Check sheet for the modelled part. Datum: model origin and axes. Units: mm. A direction names the side the tool comes from. Coordinates: 2 decimals unless noted, no trailing zeros. Loops run counter-clockwise (first coordinate to the right, second up) from the corner with the lowest first, then second, coordinate; pieces in that order, holes last. Notation, with made-up numbers: (-10.5, -16.5) - (0.5, -16.5) arc R22 ccw to (0.5, 21.5) - close; hole circle Ø4 at (6, 30.25). An arc over 180 degrees is marked (long way). Use a Markdown table: item, result. Add a question column.
1) Tool access check on faces 5 (the flat face through (30.4, 19.9, 4.5)), 6 (the flat face through (-31, 18.5, 17)). Record the directions out of +Z, -Z, +X, -X, +Y, -Y that give a thin tool (end or side, any length) a straight path to the whole face; none if there is none.
2) Sectioned sample at B-B, the plane z = 18.75. Enter the section's corners in (x, y), then the cut area to 3 significant figures.
3) Sectioned sample at A-A, the plane x = 31. Enter the section's corners in (y, z).
4) Go/stop test with flat-tipped pins: P1, Ø2, axis at x = 21, z = 5.5, coming from the +Y side; P2, Ø0.9, axis at y = -11, z = 1.5, coming from the -X side; P3, Ø2, axis at x = -3.5, z = 5.5, coming from the -Y side. Record where each tip stops, or that it passes through.
5) Sectioned sample at C-C, the plane y = 15.5. Enter the section's corners in (x, z).
6) Draft check along X on faces 1 (the cylindrical face through (-36.1, 20.02, 26.14)), 2 (the flat face through (0, 41.5, 8)), 3 (the flat face through (37, 20, 18)), 4 (the cylindrical face through (14, -15.43, 1.52)). Enter one of: pulls with the +X half, pulls with the -X half, needs draft (parallel to the pull), parting line crosses it, or undercut.
7) Sectioned sample at D-D, the plane z = 13.75. Enter the section's corners in (x, y), then the cut area to 3 significant figures.
8) Thickness scan on line 1 (X direction, y = 20.6, z = 20); line 2 (X direction, y = 5, z = 12.25); line 3 (Y direction, x = -15.5, z = 1.8). Record the ranges inside material, lowest first.
from build123d import *

# Parameters (mm, degrees)
BOSS_EXTRUDE1_DEPTH     = 3
BOSS_EXTRUDE2_DEPTH     = 27
BOSS_EXTRUDE2_2_DEPTH   = 27
BOSS_EXTRUDE3_DEPTH     = 10
SKETCH4_W               = 26
SKETCH4_H               = 17
BOSS_EXTRUDE4_DEPTH     = 7
CUT_EXTRUDE1_DEPTH      = 80.342611502
SKETCH6_R               = 2.2
CUT_EXTRUDE2_DEPTH      = 61.811183182
SKETCH7_W               = 20
SKETCH7_H               = 7
CUT_EXTRUDE3_DEPTH      = 17
SKETCH8_R               = 12
SKETCH8_R_2             = 1.5
CUT_EXTRUDE4_DEPTH      = 61.557823607
SKETCH9_R               = 2.2
CUT_EXTRUDE5_DEPTH      = 59.139917441
FILLET1_R               = 7
FILLET2_R               = 3
CHAMFER1_SIZE           = 6
CUT_EXTRUDE6_DEPTH      = 61.557823607
CUT_EXTRUDE6_DEPTH_BACK = 61.557823607
FILLET3_R               = 1


with BuildPart() as part:
    # Sketch1 → Boss-Extrude1 (new body)
    with BuildSketch(Plane.XY):
        Polygon((-13, 21.5), (-13, 41.5), (13, 41.5), (13, 21.5), (22, 21.5), (22, -21.5), (-22, -21.5), (-22, 21.5), align=None)
    extrude(amount=BOSS_EXTRUDE1_DEPTH)



with BuildPart() as body_2:
    # Sketch2 → Boss-Extrude2 (new body)
    with BuildSketch(Plane(origin=(0, 0, 0), x_dir=(-1, 0, 0), z_dir=(0, 0, -1))):
        Polygon((37, 21.5), (22, 21.5), (22, -7.5), (25, -7.5), (25, 18.5), (37, 18.5), align=None)
    extrude(amount=-BOSS_EXTRUDE2_DEPTH)


with BuildPart() as body_3:
    # Sketch2 → Boss-Extrude2 2 (new body)
    with BuildSketch(Plane(origin=(0, 0, 0), x_dir=(-1, 0, 0), z_dir=(0, 0, -1))):
        Polygon((-37, 18.5), (-37, 21.5), (-22, 21.5), (-22, -7.5), (-25, -7.5), (-25, 18.5), align=None)
    extrude(amount=-BOSS_EXTRUDE2_2_DEPTH)


with BuildPart() as part_1:
    add(part.part)

    add(body_2.part)  # Boss-Extrude3 merges body 2

    add(body_3.part)  # Boss-Extrude3 merges body 3
    # Sketch3 → Boss-Extrude3 (add)
    with BuildSketch(Plane(origin=(0, 0, 0), x_dir=(-1, 0, 0), z_dir=(0, 0, -1))):
        Polygon((-25, 21.5), (-22, 24.5), (22, 24.5), (25, 21.5), align=None)
    extrude(amount=-BOSS_EXTRUDE3_DEPTH)

    # Sketch4 → Boss-Extrude4 (add)
    with BuildSketch(Plane.XY.offset(3)):
        with Locations((0, 33)):
            Rectangle(SKETCH4_W, SKETCH4_H)
    extrude(amount=BOSS_EXTRUDE4_DEPTH)

    # Sketch5 → Cut-Extrude1 (cut, through all)
    with BuildSketch(Plane(origin=(25, 0, 0), x_dir=(0, 0, -1), z_dir=(1, 0, 0))):
        Polygon((-27, 18.5), (-3, -7.5), (-27, -7.5), align=None)
    extrude(amount=-CUT_EXTRUDE1_DEPTH, mode=Mode.SUBTRACT)

    # Sketch6 → Cut-Extrude2 (cut, through all)
    with BuildSketch(Plane.XZ.offset(-18.5)):
        with Locations(Location((31, 20, 0), (0, 0, 270))):
            Circle(SKETCH6_R)
        with Locations(Location((-31, 20, 0), (0, 0, 180))):
            Circle(SKETCH6_R)
        Polygon((25, 0), (37, 10), (37, 0), align=None)
        Polygon((-37, 0), (-25, 0), (-37, 10), align=None)
    extrude(amount=-CUT_EXTRUDE2_DEPTH, mode=Mode.SUBTRACT)

    # Sketch7 → Cut-Extrude3 (cut)
    with BuildSketch(Plane(origin=(0, 41.5, 0), x_dir=(1, 0, 0), z_dir=(0, 1, 0))):
        with Locations((0, -3.5)):
            Rectangle(SKETCH7_W, SKETCH7_H)
    extrude(amount=-CUT_EXTRUDE3_DEPTH, mode=Mode.SUBTRACT)

    # Sketch8 → Cut-Extrude4 (cut, through all)
    with BuildSketch(Plane.XY.offset(3)):
        Circle(SKETCH8_R)
        with Locations((-15.5, 15.5)):
            Circle(SKETCH8_R_2)
        with Locations((15.5, 15.5)):
            Circle(SKETCH8_R_2)
        with Locations((15.5, -15.5)):
            Circle(SKETCH8_R_2)
        with Locations((-15.5, -15.5)):
            Circle(SKETCH8_R_2)
    extrude(amount=-CUT_EXTRUDE4_DEPTH, mode=Mode.SUBTRACT)

    # Sketch9 → Cut-Extrude5 (cut, through all)
    with BuildSketch(Plane.XY.offset(10)):
        with Locations((0, 31.5)):
            Circle(SKETCH9_R)
    extrude(amount=-CUT_EXTRUDE5_DEPTH, mode=Mode.SUBTRACT)

    # Fillet1
    fillet1_edges = [part_1.edges().sort_by_distance(p)[0] for p in [
        (13, 24.5, 5),
        (-13, 24.5, 5),
    ]]
    fillet(fillet1_edges, radius=FILLET1_R)

    # Fillet2
    fillet2_edges = [part_1.edges().sort_by_distance(p)[0] for p in [
        (13, 41.5, 5),
        (-13, 41.5, 5),
        (-37, 20, 10),
        (37, 20, 10),
        (-37, 20, 27),
        (37, 20, 27),
    ]]
    fillet(fillet2_edges, radius=FILLET2_R)

    # Chamfer1
    chamfer1_edges = [part_1.edges().sort_by_distance(p)[0] for p in [
        (22, -21.5, 1.5),
        (-22, -21.5, 1.5),
    ]]
    chamfer(chamfer1_edges, length=CHAMFER1_SIZE)

    # Sketch10 → Cut-Extrude6 (cut, two sides: drawn at the far end of the back side and taken through both)
    with BuildSketch(Plane.XY.offset(3).offset(-CUT_EXTRUDE6_DEPTH_BACK)):
        Polygon((22, -7.5), (25, -4.510011911), (25, -7.5), align=None)
        Polygon((-22, -7.5), (-25, -7.5), (-25, -4.510005014), align=None)
    extrude(amount=CUT_EXTRUDE6_DEPTH + CUT_EXTRUDE6_DEPTH_BACK, mode=Mode.SUBTRACT)

    # Fillet3
    fillet3_edges = [part_1.edges().sort_by_distance(p)[0] for p in [
        (-25, 18.5, 13.5),
        (25, 18.5, 13.5),
    ]]
    fillet(fillet3_edges, radius=FILLET3_R)


solid = part_1.part
Solved:
| question | item | result |
|---|---|---|
| 1 | face 5 | -Z, +X, +Y, -Y |
| 1 | face 6 | +Z, -Z, -X, -Y |
| 2 | outline | (-37, 18.5) - (-32.81, 18.5) - (-32.81, 21.5) - (-37, 21.5) - close; (-29.19, 18.5) - (-26, 18.5) arc R1 cw to (-25, 17.5) - (-25, 9.56) - (-22, 9.56) - (-22, 21.5) - (-29.19, 21.5) - close; (22, 9.56) - (25, 9.56) - (25, 17.5) arc R1 cw to (26, 18.5) - (29.19, 18.5) - (29.19, 21.5) - (22, 21.5) - close; (32.81, 18.5) - (37, 18.5) - (37, 21.5) - (32.81, 21.5) - close |
| 2 | area | 122 mm2 |
| 3 | outline | (18.5, 5) - (21.5, 5) - (21.5, 17.8) - (18.5, 17.8) - close; (18.5, 22.2) - (21.5, 22.2) - (21.5, 27) - (18.5, 27) - close |
| 4 | P1 | stops at y = 24.5 |
| 4 | P2 | stops at x = -22 |
| 4 | P3 | stops at y = 21.5 |
| 5 | outline | (-25, 0) - (-17, 0) - (-17, 3) - (-22, 3) - (-22, 24.23) - (-25, 24.23) - close; (-14, 0) - (14, 0) - (14, 3) - (-14, 3) - close; (17, 0) - (25, 0) - (25, 24.23) - (22, 24.23) - (22, 3) - (17, 3) - close |
| 6 | face 1 | pulls with the -X half |
| 6 | face 2 | needs draft |
| 6 | face 3 | pulls with the +X half |
| 6 | face 4 | undercut |
| 7 | outline | (-37, 18.5) - (-26, 18.5) arc R1 cw to (-25, 17.5) - (-25, 4.15) - (-22, 4.15) - (-22, 21.5) - (-37, 21.5) - close; (22, 4.15) - (25, 4.15) - (25, 17.5) arc R1 cw to (26, 18.5) - (37, 18.5) - (37, 21.5) - (22, 21.5) - close |
| 7 | area | 177 mm2 |
| 8 | line 1 | x = -37 to -33.2, -28.8 to -22, 22 to 28.8, 33.2 to 37 |
| 8 | line 2 | x = -25 to -22, 22 to 25 |
| 8 | line 3 | y = -21.5 to -17, -14 to 14, 17 to 26.14 |
